from build123d import *

# Parameters (mm, degrees)
SKETCH1_R           = 9.1
BOSS_EXTRUDE1_DEPTH = 72.5
CUT_EXTRUDE2_DEPTH  = 2


with BuildPart() as part:
    # Sketch1 → Boss-Extrude1 (new body)
    with BuildSketch(Plane(origin=(0, 0, 0), x_dir=(1, 0, 0), z_dir=(0, 1, 0))):
        with Locations(Location((0, 0, 0), (0, 0, 270))):
            Circle(SKETCH1_R)
    extrude(amount=BOSS_EXTRUDE1_DEPTH)

    # Sketch3 → Cut-Extrude2 (cut)
    with BuildSketch(Plane(origin=(0, 72.5, 0), x_dir=(1, 0, 0), z_dir=(0, 1, 0))):
        with BuildLine():
            Line((-3.582051282, 6.265328291), (-1.09140625, 6.265328291))
            add(Edge.make_bspline(
                [(-1.09140625, 6.265328291), (-0.920098105, 6.265139982), (-0.591864091, 6.264779173), (-0.121183746, 6.253839953), (0.30629728, 6.239228813), (0.689657234, 6.218974515), (1.030075647, 6.195038316), (1.326012134, 6.16146663), (1.57979281, 6.126413557), (1.731853355, 6.090775882), (1.801201923, 6.074523003)],
                knots=[0, 0, 0, 0, 1.415646017, 2.712440637, 3.8905458, 4.950247383, 5.884950622, 6.709939814, 7.411656543, 8, 8, 8, 8], degree=3))
            add(Edge.make_bspline(
                [(1.801201923, 6.074523003), (1.888989889, 6.050494785), (2.062497206, 6.003004544), (2.312509562, 5.907886176), (2.550376373, 5.795102319), (2.776913742, 5.666564023), (2.989337872, 5.516756405), (3.190818078, 5.351752134), (3.379576292, 5.167741586), (3.554551057, 4.966788615), (3.715241608, 4.752266711), (3.853597886, 4.520973477), (3.969448109, 4.276802176), (4.068810266, 4.019922646), (4.140323801, 3.748177758), (4.194196837, 3.463455687), (4.228391143, 3.165786954), (4.231666153, 2.962369721), (4.233333333, 2.858817875)],
                knots=[0, 0, 0, 0, 0.999701418, 1.975846123, 2.934577507, 3.890451536, 4.834027766, 5.787354733, 6.749476667, 7.726910423, 8.712836071, 9.690891519, 10.682875813, 11.679750201, 12.712814741, 13.765529915, 14.8625177, 16, 16, 16, 16], degree=3))
            add(Edge.make_bspline(
                [(4.233333333, 2.858817875), (4.231804164, 2.754395656), (4.22881224, 2.550086532), (4.192902862, 2.251190987), (4.144533309, 1.965555685), (4.070158291, 1.693813965), (3.972746848, 1.437579598), (3.858475685, 1.192936842), (3.720649732, 0.964047747), (3.56228135, 0.750081349), (3.386108422, 0.55083681), (3.192876332, 0.367757984), (2.983365185, 0.201916527), (2.758240819, 0.052940652), (2.51530851, -0.075714991), (2.258252696, -0.19094864), (1.984839053, -0.287726489), (1.795636217, -0.338635569), (1.699439103, -0.364519465)],
                knots=[0, 0, 0, 0, 1.121902311, 2.195077645, 3.232258892, 4.234102512, 5.217864754, 6.176164875, 7.132989551, 8.084763148, 9.034132444, 9.988522005, 10.94243251, 11.903244335, 12.886203696, 13.894208494, 14.929344452, 16, 16, 16, 16], degree=3))
            add(Edge.make_bspline(
                [(1.699439103, -0.364519465), (1.619874205, -0.381439425), (1.445503106, -0.418520501), (1.158328085, -0.459916902), (0.823971971, -0.495250481), (0.442891126, -0.52174318), (0.015427614, -0.544423089), (-0.458649805, -0.562450172), (-0.980271743, -0.572355642), (-1.344113114, -0.572866519), (-1.534074519, -0.573133247)],
                knots=[0, 0, 0, 0, 0.601384939, 1.31797006, 2.144135048, 3.087295005, 4.142315834, 5.309527816, 6.595305764, 8, 8, 8, 8], degree=3))
            Line((-1.534074519, -0.573133247), (-2.442307692, -0.573133247))
            Line((-2.442307692, -0.573133247), (-2.442307692, -6.434671709))
            Line((-2.442307692, -6.434671709), (-3.582051282, -6.434671709))
            Line((-3.582051282, -6.434671709), (-3.582051282, 6.265328291))
        make_face()
        with BuildLine():
            Line((-2.442307692, 4.962764189), (-2.442307692, 0.729430855))
            Line((-2.442307692, 0.729430855), (-0.218790064, 0.70144608))
            add(Edge.make_bspline(
                [(-0.218790064, 0.70144608), (-0.110223476, 0.701389969), (0.099362084, 0.701281648), (0.402116379, 0.715742316), (0.683001508, 0.732435678), (0.941154681, 0.756877457), (1.176692272, 0.79142602), (1.39000702, 0.826302898), (1.579444875, 0.876759499), (1.801147692, 0.944697493), (2.048192982, 1.06056727), (2.316952372, 1.228751156), (2.544719928, 1.443129726), (2.741817748, 1.684167857), (2.898230505, 1.952316127), (3.012733677, 2.239223411), (3.080011591, 2.541947322), (3.089032922, 2.749095712), (3.093589744, 2.853729734)],
                knots=[0, 0, 0, 0, 1.160613943, 2.240541288, 3.23993089, 4.169200891, 5.011653406, 5.7853311, 6.478053781, 7.106038997, 8.262395093, 9.384106736, 10.481365981, 11.59014053, 12.70357646, 13.786202915, 14.881775077, 16, 16, 16, 16], degree=3))
            add(Edge.make_bspline(
                [(3.093589744, 2.853729734), (3.089008141, 2.955832339), (3.079900481, 3.158799683), (3.012206349, 3.456265472), (2.898453124, 3.740149313), (2.740767767, 4.004937366), (2.54939281, 4.245108169), (2.326963765, 4.453740601), (2.074004216, 4.621459351), (1.838697778, 4.729711545), (1.62968776, 4.795806973), (1.44814322, 4.842052537), (1.243162773, 4.878975451), (1.014679687, 4.908873075), (0.76446489, 4.934467063), (0.490368719, 4.951833323), (0.193429499, 4.961998607), (-0.012711715, 4.962502816), (-0.119571314, 4.962764189)],
                knots=[0, 0, 0, 0, 1.120700087, 2.227813068, 3.331159281, 4.466773991, 5.599788987, 6.693661531, 7.80175334, 8.91857717, 9.525282508, 10.207424825, 10.974604443, 11.810962634, 12.737642355, 13.736264703, 14.826523623, 16, 16, 16, 16], degree=3))
            Line((-0.119571314, 4.962764189), (-2.442307692, 4.962764189))
        make_face(mode=Mode.SUBTRACT)
    extrude(amount=-CUT_EXTRUDE2_DEPTH, mode=Mode.SUBTRACT)


solid = part.part
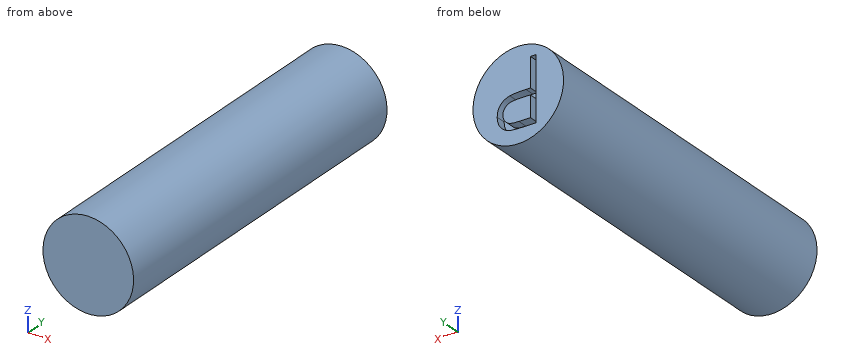
Can you work these out from the model? Positions are in its coordinate system, mm. Give positions to 0.01 mm unless a question says otherwise; leave off trailing zeros. Loops run counter-clockwise (first coordinate to the right, second up) from the corner with the lowest first, then second, coordinate; pieces in that order, holes last. Notation, with made-up numbers: M 6.5,23.25 L 10.5,23.25 A11 cw 10.5,31.25 Z; hole C -37,-15.75 d3. An arc over 180 degrees is marked long. One line per item, written item: value.
1) Imagine slicing it at C-C on x = -8. Write out the boundary of the cut face in (y, z), and give its area (3 significant figures).
Geometry check:
outline: M 0,-4.34 L 72.5,-4.34 L 72.5,4.34 L 0,4.34 Z
area: 629 mm²
2) Please list where these lines run through material, in increasing order: line 1 (Y direction, x = -2.75, z = 1); line 2 (X direction, y = 26, z = 0.5); line 3 (X direction, y = 39.5, z = 8).
Geometry check:
line 1: y = 0 to 70.5
line 2: x = -9.09 to 9.09
line 3: x = -4.34 to 4.34
3) Imagine slicing it at A-A on z = 5.5. Write out the boundary of the cut face in (x, y).
Geometry check:
outline: M -7.25,0 L 7.25,0 L 7.25,72.5 L -2.44,72.5 L -2.44,70.5 L -3.58,70.5 L -3.58,72.5 L -7.25,72.5 Z
4) I'm going to push flat-ended pins straight in: pin 1 (1 mm diameter, centred on y = 16.5, z = -6, fed in from -X); pin 2 (1 mm diameter, centred on x = -1, y = 71.5, fed in from -Z); pin 3 (3 mm diameter, centred on x = 3, y = 46.5, fed in from +Z). Where does each tip first touch, or does it pass through?
Geometry check:
pin 1: stops at x = -7.25
pin 2: stops at z = -9.09
pin 3: stops at z = 8.98
5) Imagine slicing it at B-B on y = 67.5. Write out the boundary of the cut face in (x, z).
Geometry check:
outline: C 0,0 d18.2
6) Imagine slicing it at D-D on z = 2.75. Write out the boundary of the cut face in (x, y), and give its area (3 significant figures).
Geometry check:
outline: M -8.67,0 L 8.67,0 L 8.67,72.5 L -2.44,72.5 L -2.44,70.5 L -3.58,70.5 L -3.58,72.5 L -8.67,72.5 Z
area: 1,260 mm²
